Source: CAD feature listing. Evaluate the final solid. Frame: model axes, mm. Face numbers are marked on the shaded views. Give positions to 0.01 mm unless a question says otherwise; leave off trailing zeros. Loops run counter-clockwise (first coordinate to the right, second up) from the corner with the lowest first, then second, coordinate; pieces in that order, holes last. Notation, with made-up numbers: M 74.5,38.5 L 130.5,38.5 A29 cw 130.5,75.5 Z; hole C 49,-14 d11. An arc over 180 degrees is marked long. Answer in a Markdown table with one row per item.
```python
from build123d import *

# Parameters (mm, degrees)
F0_R     = 13
F1_DEPTH = 5
F2_SIZE  = 1
F3_R     = 2


with BuildPart() as f1:
    # F0 (on Top) → F1 (new body, symmetric)
    with BuildSketch(Plane.XY):
        Polygon((-10.5591686686, -17.9026243056), (10.2245431088, -18.0958204627), (20.7837117774, -0.193196157), (10.5591686686, 17.9026243056), (-10.2245431088, 18.0958204627), (-20.7837117774, 0.193196157), align=None)
        Circle(F0_R, mode=Mode.SUBTRACT)
    extrude(amount=F1_DEPTH, both=True)

    # F2
    f2_edges = [f1.edges().sort_by_distance(p)[0] for p in [
        (-15.67144, -8.854714, 5),
        (-0.167313, -17.999222, 5),
        (15.504127, -9.144508, 5),
        (15.67144, 8.854714, 5),
        (0.167313, 17.999222, 5),
        (-15.504127, 9.144508, 5),
        (-13, 0, 5),
        (-15.67144, -8.854714, -5),
        (-0.167313, -17.999222, -5),
        (15.504127, -9.144508, -5),
        (15.67144, 8.854714, -5),
        (0.167313, 17.999222, -5),
        (-15.504127, 9.144508, -5),
        (-13, 0, -5),
    ]]
    chamfer(f2_edges, length=F2_SIZE)

    # F3
    f3_edges = [f1.edges().sort_by_distance(p)[0] for p in [
        (10.559169, 17.902624, 0),
        (-10.224543, 18.09582, 0),
        (-20.783712, 0.193196, 0),
        (-10.559169, -17.902624, 0),
        (10.224543, -18.09582, 0),
        (20.783712, -0.193196, 0),
    ]]
    fillet(f3_edges, radius=F3_R)


solid = f1.part
```
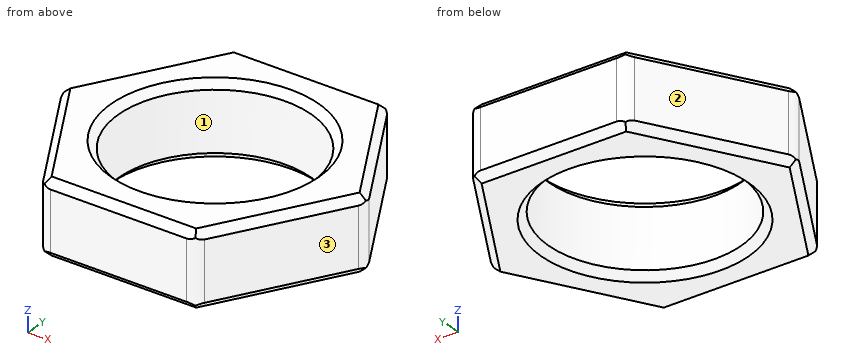
Q1. Ray query, probe 1 along Y at (x, z) = (7.5, -3.75); probe 2 along Y at (x, z) = (10, 0.25); probe 3 along X at (y, z) = (-12, 1.5). Return the intervals inside material, ascending. Write a range as from..to.
Values follow:
| item | result |
|---|---|
| probe 1 | -18.07..-10.62, 10.62..17.93 |
| probe 2 | -17.87..-8.31, 8.31..17.82 |
| probe 3 | -13.89..-5, 5..13.82 |
Q2. Section query C-C (y = -15). Output: boundary loops of the cut face in (x, z), plus the area to 3 significant figures.
Values follow:
| item | result |
|---|---|
| outline | M -12.2,-4 L -11.05,-5 L 10.89,-5 L 12.05,-4 L 12.05,4 L 10.89,5 L -11.05,5 L -12.2,4 Z |
| area | 240 mm^2 |
Q3. Contact query for flat-ended pins moving along their axis: pin 1 Ø6 at (x, z) = (-3.5, -1.5) entering from -Y; pin 2 Ø2 at (y, z) = (14, 0.5) entering from -X; pin 3 Ø3 at (x, z) = (-16.5, -2) entering from +Y; pin 4 Ø21 at (x, y) = (0, 0) entering from -Z. Output: stop coordinate, or through.
Values follow:
| item | result |
|---|---|
| pin 1 | y = -18 |
| pin 2 | x = -13.23 |
| pin 3 | y = 10 |
| pin 4 | through |
Q4. Mould query, pull axis Y, two halves, no side actions, for the marked faces 1, 2 and 3. Classes: +Y half, -Y half, draft (parallel to the pull), parting line (faces both ways), or undercut.
Values follow:
| item | result |
|---|---|
| face 1 | undercut |
| face 2 | +Y half |
| face 3 | -Y half |
Q5. Section query B-B (z = 0.25). Output: boundary loops of the cut face in (x, y), plus the area to 3 significant figures.
Values follow:
| item | result |
|---|---|
| outline | M -20.22,-0.81 L -11.13,-16.9 A2 ccw -9.4,-17.91 L 9.07,-18.09 A2 ccw 10.81,-17.1 L 20.2,-1.19 A2 ccw 20.22,0.81 L 11.13,16.9 A2 ccw 9.4,17.91 L -9.07,18.09 A2 ccw -10.81,17.1 L -20.2,1.19 A2 ccw Z; hole C 0,0 d26 |
| area | 590 mm^2 |
Q6. Section query A-A (x = 0). Output: boundary loops of the cut face in (y, z).
Values follow:
| item | result |
|---|---|
| outline | M -18,-4 L -17,-5 L -14,-5 L -13,-4 L -13,4 L -14,5 L -17,5 L -18,4 Z; M 13,-4 L 14,-5 L 17,-5 L 18,-4 L 18,4 L 17,5 L 14,5 L 13,4 Z |
Q7. Section query D-D (x = 16). Output: boundary loops of the cut face in (y, z).
Values follow:
| item | result |
|---|---|
| outline | M -8.3,-4 L -6.34,-5 L 6.24,-5 L 8.27,-4 L 8.27,4 L 6.24,5 L -6.34,5 L -8.3,4 Z |
